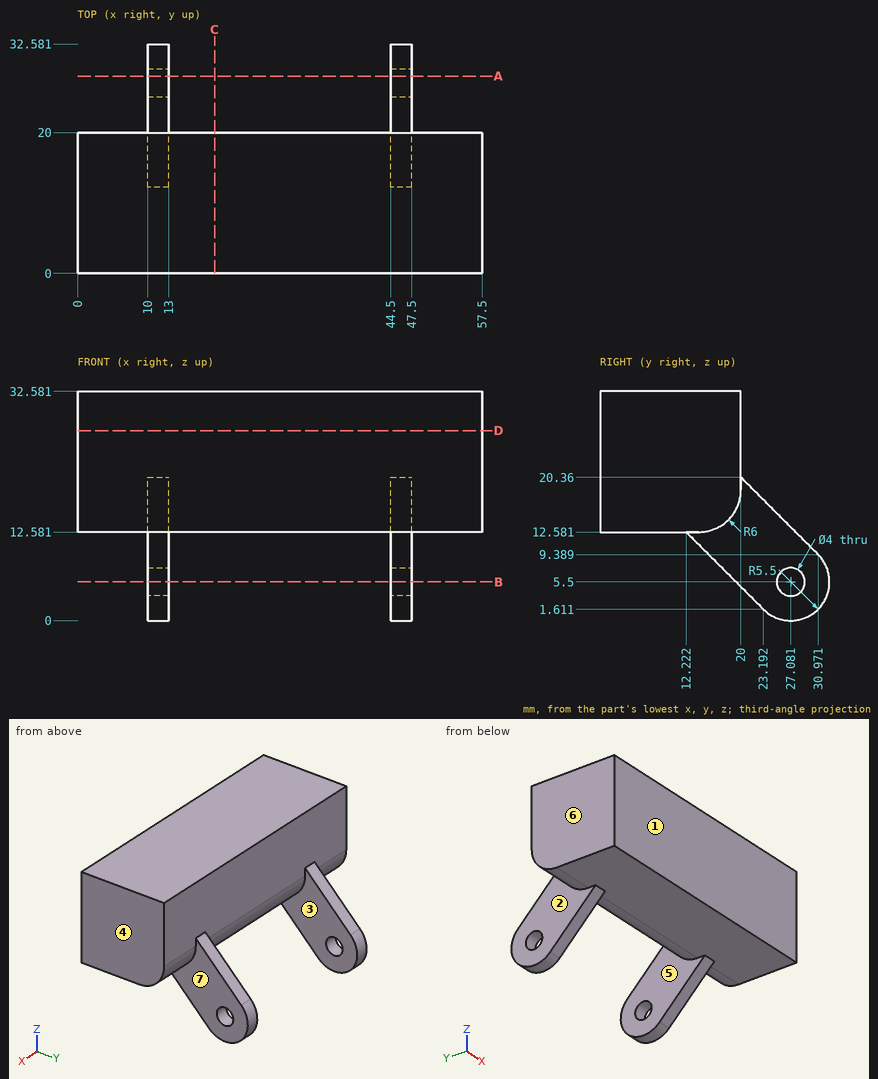
Here's the drawing with two shaded views (mm, measured from the low corner). I have some questions. A direction names the side the tool comes from. Give positions to 0.01 mm unless a question says otherwise; leave off trailing zeros. Order: outer loops, then holes, each group sorted by start corner. A loop starts at its lowest first (then second) coordinate and runs counter-clockwise, first axis right, second up.
Q1. For the marked faces 5, 6 and 7, which set-ups out of +Z, -Z, +X, -X, +Y, -Y let a thin tool reach every point of the face, with its end or its side?
Q2. Suppose I cut it at B-B, the plane z = 5.5. Write out the boundary of the cut face in (x, y).
Q3. Suppose I cut it at C-C, the plane x = 19.5. Write out the boundary of the cut face in (y, z).
Q4. We'd pull the mould along X, two halves only. Please class the marked faces 1, 2, 3 and 4: +X half, -X half, draft (parallel to the pull), parting line (faces both ways), or undercut.
Q5. I'm going to push flat-ended pins straight in: P1, Ø4.5, axis at y = 27.08, z = 5.5, coming from the +X side; P2, Ø1.5, axis at x = 41, y = 17.5, coming from the -Z side; P3, Ø12, axis at x = 25, z = 23, coming from the +Y side. Where does each tip first touch, or does it pass through?
Q6. If I drill on line 1 along X through (y, z) = (14.5, 12.5); line 2 along Z through (x, y) = (2, 8); line 3 along Y through (x, z) = (10.8, 5.5) (1 decimal), over which ranges is the centre line in solid material (lowest first)?
Q7. Suppose I cut it at D-D, the plane z = 27. Write out the boundary of the cut face in (x, y).
Q8. Suppose I cut it at A-A, the plane y = 28. Write out the boundary of the cut face in (x, z).
Solution:
1. face 5: -Z, +Y
1. face 6: +Z, -Z, -X, +Y, -Y
1. face 7: -Z, +X, +Y
2. outline: (10, 19.3) - (13, 19.3) - (13, 25.08) - (10, 25.08) - close; (10, 29.08) - (13, 29.08) - (13, 32.58) - (10, 32.58) - close; (44.5, 19.3) - (47.5, 19.3) - (47.5, 25.08) - (44.5, 25.08) - close; (44.5, 29.08) - (47.5, 29.08) - (47.5, 32.58) - (44.5, 32.58) - close
3. outline: (0, 12.58) - (14, 12.58) arc R6 ccw to (20, 18.58) - (20, 32.58) - (0, 32.58) - close
4. face 1: draft
4. face 2: -X half
4. face 3: undercut
4. face 4: +X half
5. P1: stops at x = 47.5
5. P2: stops at z = 13.25
5. P3: stops at y = 20
6. line 1: x = 10 to 13, 44.5 to 47.5
6. line 2: z = 12.58 to 32.58
6. line 3: y = 19.3 to 25.1, 29.1 to 32.6
7. outline: (0, 0) - (57.5, 0) - (57.5, 20) - (0, 20) - close
8. outline: (10, 0.08) - (13, 0.08) - (13, 3.72) - (10, 3.72) - close; (10, 7.28) - (13, 7.28) - (13, 12.36) - (10, 12.36) - close; (44.5, 0.08) - (47.5, 0.08) - (47.5, 3.72) - (44.5, 3.72) - close; (44.5, 7.28) - (47.5, 7.28) - (47.5, 12.36) - (44.5, 12.36) - close
